Can you work these out from the model? Positions are in its coordinate system, mm. Face numbers are marked on the shaded views. Round coordinates to 2 decimals unless told otherwise and drop trailing zeros. Write each loop counter-clockwise with the first axis right and the second up, starting at its lowest first coordinate (ties: lowest second). Pieces come first, ordered by that corner, then holes. Notation, with made-up numbers: M 51,-4.75 L 98,-4.75 A20 ccw 98,9.25 Z; hole C 62.25,-30 d5. An arc over 180 degrees is marked long. Answer in a Markdown table with one row per item. Add a question column.
(1) If I drill on probe 1 along X at (y, z) = (-56, 52); probe 2 along X at (y, z) = (-23, 81.5); probe 3 along Z at (x, y) = (36, -49), over which ranges is the centre line in solid material (lowest first)?
(2) Suppose I cut it at B-B, the plane z = 27. Write out the boundary of the cut face in (x, y), then the cut area to 3 significant figures.
(3) Suppose I cut it at C-C, the plane x = 13.5. Write out the boundary of the cut face in (y, z), then the cut area to 3 significant figures.
(4) Suppose I cut it at A-A, the plane y = -23. Write out the boundary of the cut face in (x, z), then the cut area to 3 significant figures.
(5) If we mould it in two halves opening along X, with no side actions, what happens to the marked faces 1, 2, 3 and 4? For each: released by +X, released by -X, zero draft, split by the parting line, or undercut.
(6) I'm going to push flat-ended pins straight in: pin 1 (1 mm diameter, centred on x = 30.5, y = -58, fed in from +Z); pin 2 (5 mm diameter, centred on x = 44.5, z = 71.5, fed in from +Y). Where does each tip first touch, or does it pass through?
(7) Suppose I cut it at D-D, the plane y = -121. Write out the boundary of the cut face in (x, z), then the cut area to 3 significant figures.
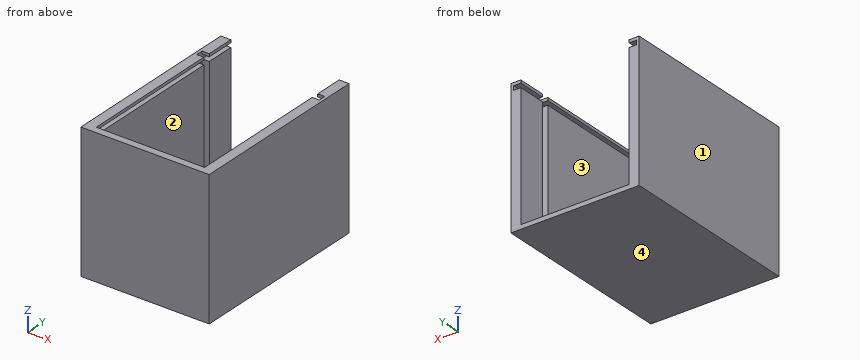
from build123d import *

# Parameters (mm, degrees)
SKETCH_1_W           = 96
SKETCH_1_H           = 130
EXTRUDE_1_DEPTH      = 96
SKETCH_3_W           = 76
SKETCH_3_H           = 93
CUT_EXTRUDE_1_DEPTH  = 130
SKETCH_8_W           = 86
SKETCH_8_H           = 125
CUT_EXTRUDE_5_DEPTH  = 3
SKETCH_10_W          = 91
SKETCH_10_H          = 5
CUT_EXTRUDE_7_DEPTH  = 86
SKETCH_15_W          = 96
SKETCH_15_H          = 130
CUT_EXTRUDE_10_DEPTH = 3
SKETCH_16_W          = 96
SKETCH_16_H          = 130
CUT_EXTRUDE_11_DEPTH = 3


with BuildPart() as part:
    # 草圖1 → 填料-伸長1 (new body)
    with BuildSketch(Plane.XY):
        with Locations((48, -65)):
            Rectangle(SKETCH_1_W, SKETCH_1_H)
    extrude(amount=EXTRUDE_1_DEPTH)

    # 草圖3 → 除料-伸長1 (cut)
    with BuildSketch(Plane(origin=(0, -125, 0), x_dir=(-1, 0, 0), z_dir=(0, -1, 0))):
        with Locations((-48, -49.5)):
            Rectangle(SKETCH_3_W, SKETCH_3_H)
    extrude(amount=-CUT_EXTRUDE_1_DEPTH, mode=Mode.SUBTRACT)

    # 草圖8 → 除料-伸長5 (cut)
    with BuildSketch(Plane.XY.offset(94)):
        with Locations((48, -62.5)):
            Rectangle(SKETCH_8_W, SKETCH_8_H)
    extrude(amount=-CUT_EXTRUDE_5_DEPTH, mode=Mode.SUBTRACT)

    # 草圖10 → 除料-伸長7 (cut)
    with BuildSketch(Plane.ZY.offset(-5)):
        with Locations((50.5, -22.5)):
            Rectangle(SKETCH_10_W, SKETCH_10_H)
    extrude(amount=-CUT_EXTRUDE_7_DEPTH, mode=Mode.SUBTRACT)

    # 草圖15 → 除料-伸長10 (cut)
    with BuildSketch(Plane.ZY):
        with Locations((48, -65)):
            Rectangle(SKETCH_15_W, SKETCH_15_H)
    extrude(amount=-CUT_EXTRUDE_10_DEPTH, mode=Mode.SUBTRACT)

    # 草圖16 → 除料-伸長11 (cut)
    with BuildSketch(Plane(origin=(96, 0, 0), x_dir=(0, 0, -1), z_dir=(1, 0, 0))):
        with Locations((-48, -65)):
            Rectangle(SKETCH_16_W, SKETCH_16_H)
    extrude(amount=-CUT_EXTRUDE_11_DEPTH, mode=Mode.SUBTRACT)


solid = part.part
Calculated:
| question | item | result |
|---|---|---|
| 1 | probe 1 | 3 to 10, 86 to 93 |
| 1 | probe 2 | 3 to 5, 91 to 93 |
| 1 | probe 3 | 0 to 3 |
| 2 | outline | M 3,-130 L 93,-130 L 93,0 L 86,0 L 86,-20 L 91,-20 L 91,-25 L 86,-25 L 86,-125 L 10,-125 L 10,-25 L 5,-25 L 5,-20 L 10,-20 L 10,0 L 3,0 Z |
| 2 | area | 2,150 mm² |
| 3 | outline | M -130,0 L 0,0 L 0,3 L -125,3 L -125,96 L -130,96 Z |
| 3 | area | 855 mm² |
| 4 | outline | M 3,0 L 93,0 L 93,96 L 91,96 L 91,5 L 86,5 L 86,3 L 10,3 L 10,5 L 5,5 L 5,96 L 3,96 Z |
| 4 | area | 662 mm² |
| 5 | face 1 | released by -X |
| 5 | face 2 | undercut |
| 5 | face 3 | undercut |
| 5 | face 4 | zero draft |
| 6 | pin 1 | z = 3 |
| 6 | pin 2 | y = -125 |
| 7 | outline | M 3,0 L 93,0 L 93,96 L 86,96 L 86,94 L 91,94 L 91,91 L 86,91 L 86,3 L 10,3 L 10,91 L 5,91 L 5,94 L 10,94 L 10,96 L 3,96 Z |
| 7 | area | 1,540 mm² |
